Autodesk Inventor part; units mm, degrees
ref_plane "YZ Plane" through (0, 0, 0) normal (1, 0, 0) x (0, 1, 0)
ref_plane "XZ Plane" through (0, 0, 0) normal (0, 1, 0) x (-1, 0, 0)
ref_plane "XY Plane" through (0, 0, 0) normal (0, 0, 1) x (1, 0, 0)
sketch "Sketch1" plane through (0, 0, 0) normal (0, 0, 1) x (1, 0, 0)
  line L0 (0, 0) -> (50.8, 0)
  line L1 (50.8, 0) -> (50.8, 50.8)
  line L2 (50.8, 50.8) -> (0, 50.8)
  line L3 (0, 50.8) -> (0, 0)
  line L4 (3.175, 3.175) -> (47.625, 3.175)
  line L5 (47.625, 3.175) -> (47.625, 47.625)
  line L6 (47.625, 47.625) -> (3.175, 47.625)
  line L7 (3.175, 47.625) -> (3.175, 3.175)
  dimension "d0" = 50.8
  dimension "d1" = 50.8
  dimension "d2" = 44.45
  dimension "d3" = 44.45
  dimension "d4" = 3.175
  dimension "d5" = 3.175
extrude "Extrusion1" add sketch "Sketch1" along normal blind 736.6
sketch "Sketch2" plane through (50.8, 0, 0) normal (1, 0, 0) x (0, 0, -1)
  line L0 (-736.6, 50.8) -> (-711.2, 50.8)
  line L1 (-711.2, 50.8) -> (-711.2, 25.4)
  line L2 (-711.2, 25.4) -> (-736.6, 25.4)
  line L3 (-736.6, 25.4) -> (-736.6, 50.8)
  line L4 (0, 50.8) -> (-25.4, 50.8)
  line L5 (-25.4, 50.8) -> (-25.4, 25.4)
  line L6 (-25.4, 25.4) -> (0, 25.4)
  line L7 (0, 25.4) -> (0, 50.8)
  line L8 (0, 0) -> (-736.6, 0)
  line L9 (-736.6, 25.4) -> (-692.6059, 0)
  line L10 (0, 25.4) -> (-43.9941, 0)
  line L11 (0, 0) -> (0, 50.8)
  line L12 (-736.6, 0) -> (-736.6, 50.8)
  line L13 (-43.9941, 0) -> (0, 0)
  line L14 (0, 25.4) -> (0, 0)
  line L15 (-736.6, 25.4) -> (-736.6, 0)
  line L16 (-692.6059, 0) -> (-736.6, 0)
  line L17 (0, 50.8) -> (-736.6, 50.8)
  line L18 (-736.6, 25.4) -> (0, 25.4) construction
  line L19 (-368.3, 50.8) -> (-368.3, 0) construction
  circle A0 centre (-368.3, 23.8125) radius 14.2875
  circle A1 centre (-73.3171, 26.9875) radius 14.2875
  circle A2 centre (-663.2829, 26.9875) radius 14.2875
  point P0 (-402.9207, 40.0955)
  point P1 (-399.8027, 21.0564)
  point P2 (-338.5841, 34.6282)
  point P3 (-330.0412, 23.8125)
  point P4 (-404.8552, 8.9725)
  point P5 (-428.3922, 43.2675)
  dimension "d8" = 25.4
  dimension "d9" = 25.4
  dimension "d10" = 25.4
  dimension "d11" = 25.4
  dimension "d14" = 30
  dimension "d15" = 30
  dimension "d18" = 28.575
  dimension "d19" = 1.5875
  dimension "d22" = 295
  dimension "d23" = 28.575
  dimension "d24" = 28.575
  dimension "d25" = 295
  dimension "d26" = 1.5875
  dimension "d27" = 1.5875
extrude "Extrusion2" cut sketch "Sketch2" against normal up to surface (47.625 mm away) contours L0 L1 L2 L3 | L4 L7 L6 L5
extrude "Extrusion3" cut sketch "Sketch2" against normal through all contours L9 L8 L12 | L10 L11 L8
extrude "Extrusion4" cut sketch "Sketch2" against normal through all contours A0 | A1 | A2
hole "Hole1" at (50.8, 40.0955, 402.9207) at (50.8, 8.9725, 404.8552) at (50.8, 23.8125, 330.0412) at (50.8, 43.2675, 428.3922) direction (-1, 0, 0) diameter 9.1281 depth 3.175 tip angle 118
hole "Hole2" at (50.8, 21.0564, 399.8027) at (50.8, 34.6282, 338.5841) direction (-1, 0, 0) diameter 6.5278 depth 25.4 tip angle 118
sketch "Sketch3" plane through (3.175, 47.625, 711.2) normal (1, 0, 0) x (0, 0, -1)
  circle A0 centre (311.3973, -26.5686) radius 3.2639
  circle A1 centre (372.6159, -12.9968) radius 3.2639
  point P0 (711.2, -47.625)
hole "Hole3" at (3.175, 21.0564, 399.8027) at (3.175, 34.6282, 338.5841) direction (-1, 0, 0) diameter 10.3188 end through all
equation "\"d8\" = d9"
equation "\"d9\" = d11"
equation "\"d11\" = d10"
equation "\"d15\" = d14"
equation "\"d22\" = d25"
equation "\"d23\" = d18"
equation "\"d24\" = d18"
properties part number "Tube - left"
Work out the finished part from the listing and answer in its coordinate system (mm). A direction names the side the tool comes from. Round coordinates to 2 decimals unless told otherwise and drop trailing zeros. Write each loop counter-clockwise with the first axis right and the second up, starting at its lowest first coordinate (ties: lowest second). Pieces come first, ordered by that corner, then holes. Notation, with made-up numbers: (62, 20) -> (94, 20) arc R14 cw to (94, 32) -> close; hole circle Ø4 at (-24, 5). An arc over 180 degrees is marked (long way). Write each question's results on one line, items separated by ' | '.
Item 1: A cutting plane is placed at B-B, the plane x = 38.5. Determine the outline of the cut face in (y, z) (3 decimals), plus the area to 3 significant figures.
Result set:
outline: (0, 43.994) -> (3.175, 38.495) -> (3.175, 698.105) -> (0, 692.606) -> close; (47.625, 25.4) -> (50.8, 25.4) -> (50.8, 711.2) -> (47.625, 711.2) -> close | area: 4,250 mm^2
Item 2: Find the intervals of material crossed by line 1 along Y through (x, z) = (8.5, 272.5) (3 decimals); line 2 along Y through (x, z) = (2, 368), in increasing order. Write a range as [from, to].
Result set:
line 1: [0, 3.175], [47.625, 50.8] | line 2: [0, 9.53], [38.1, 50.8]
Item 3: Which of the six approach directions +Z, -Z, +X, -X, +Y, -Y give full straight-line access (tool end or side, diameter ignored) to faces 4 (the face through (49.235, 27.616, 677.557)), 5 (the face through (34, 49, 25.4)), 6 (the face through (47.625, 40, 363)), 7 (the face through (34, 49, 711.2))?
Result set:
face 4: +X, -X | face 5: -Z, +X, +Y | face 6: +Z, -Z | face 7: +Z, +X, +Y
Item 4: The mould has two halves that part along X. Classify faces 1 (the face through (0, 43, 363)), 2 (the face through (25, 3.175, 364)), 3 (the face through (1.61, 39.035, 65.636)): +X half, -X half, draft (parallel to the pull), parting line (faces both ways), or undercut.
Result set:
face 1: -X half | face 2: undercut | face 3: draft
Item 5: Flat-ended cylindrical pins translate along their axes: P1, Ø8, axis at y = 43.27, z = 428.39, coming from the +X side (3 decimals); P2, Ø1.6, axis at x = 49.5, z = 718, coming from the +Y side; P3, Ø20.5, axis at x = 17, y = 41.5, coming from the +Z side; P4, Ø1.5, axis at x = 38.5, y = 45, coming from the +Z side. Find the tip coordinate at first contact, or state that the pin passes through.
Result set:
P1: x = 3.175 | P2: y = 25.4 | P3: z = 711.2 | P4: through
Item 6: A cutting plane is placed at A-A, the plane z = 368.3. Determine the outline of the cut face in (x, y) (3 decimals).
Result set:
outline: (0, 0) -> (50.8, 0) -> (50.8, 9.525) -> (47.625, 9.525) -> (47.625, 3.175) -> (3.175, 3.175) -> (3.175, 9.525) -> (0, 9.525) -> close; (0, 38.1) -> (3.175, 38.1) -> (3.175, 47.625) -> (47.625, 47.625) -> (47.625, 38.1) -> (50.8, 38.1) -> (50.8, 50.8) -> (0, 50.8) -> close
